The drawing under review shows one solid part. Ordinate dimensions are in mm from its lowest x, y, z. Round coordinates to 2 decimals unless told otherwise and drop trailing zeros. Order: outer loops, then holes, each group sorted by start corner. A loop starts at its lowest first (then second) coordinate and runs counter-clockwise, first axis right, second up. Notation, with made-up numbers: M -11.5,-39 L -0.5,-39 A18 ccw -0.5,-4 Z; hole C -6,86 d4. An arc over 180 degrees is marked long. Answer as a JSON object with one key per item and string values. Group by question number.
1. Add section A-A on z = 10. State the section outline as (x, y) points (1 decimal).
2. Add section C-C on y = 7. State the section outline as (x, z) points, and give its area (3 significant figures).
3. To check wall thickness, follow probe 1 along Y at (x, z) = (27.5, 8.25); probe 2 along X at (y, z) = (17, 4.25); probe 3 along X at (y, z) = (23.5, 12) (1 decimal). State the ranges of each line that lie inside material, in increasing order. Write a range as [from, to].
4. Add section B-B on x = 42. State the section outline as (y, z) points.
5. Clearance check with flat-ended pins moving along their axes: P1, Ø6, axis at x = 39.5, z = 11.5, coming from the -Y side (1 decimal); P2, Ø5, axis at x = 21, z = 6, coming from the +Y side (1 decimal); P3, Ø4, axis at y = 11.5, z = 4.5, coming from the +X side (1 decimal). State where each tip first meets the part, or that it passes through.
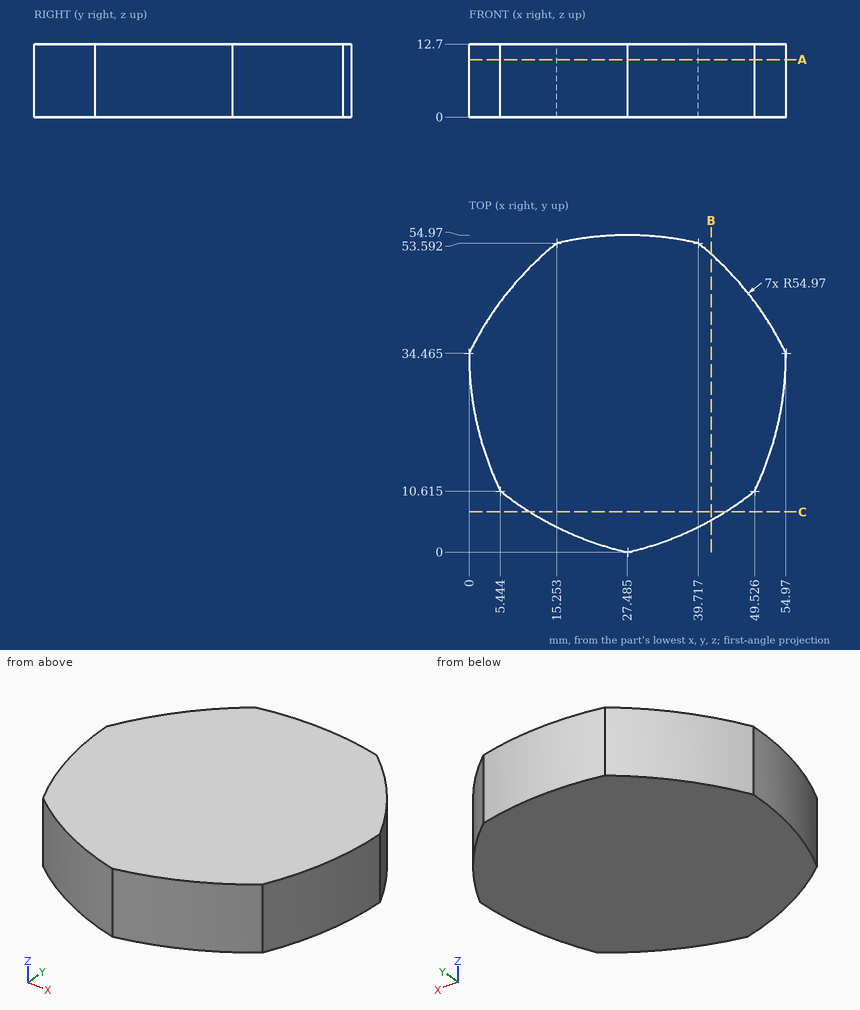
Recorded:
{
 "1": {"outline": "M 0,34.5 A55 ccw 5.4,10.6 A55 ccw 27.5,0 A55 ccw 49.5,10.6 A55 ccw 55,34.5 A55 ccw 39.7,53.6 A55 ccw 15.3,53.6 A55 ccw Z"},
 "2": {"outline": "M 10.55,0 L 44.42,0 L 44.42,12.7 L 10.55,12.7 Z", "area": "430 mm²"},
 "3": {"probe 1": "y = [0, 54.97]", "probe 2": "x = [2.85, 52.12]", "probe 3": "x = [1.1, 53.9]"},
 "4": {"outline": "M 5.57,0 L 51.67,0 L 51.67,12.7 L 5.57,12.7 Z"},
 "5": {"P1": "stops at y = 2.9", "P2": "stops at y = 54.8", "P3": "stops at x = 50.8"}
}
